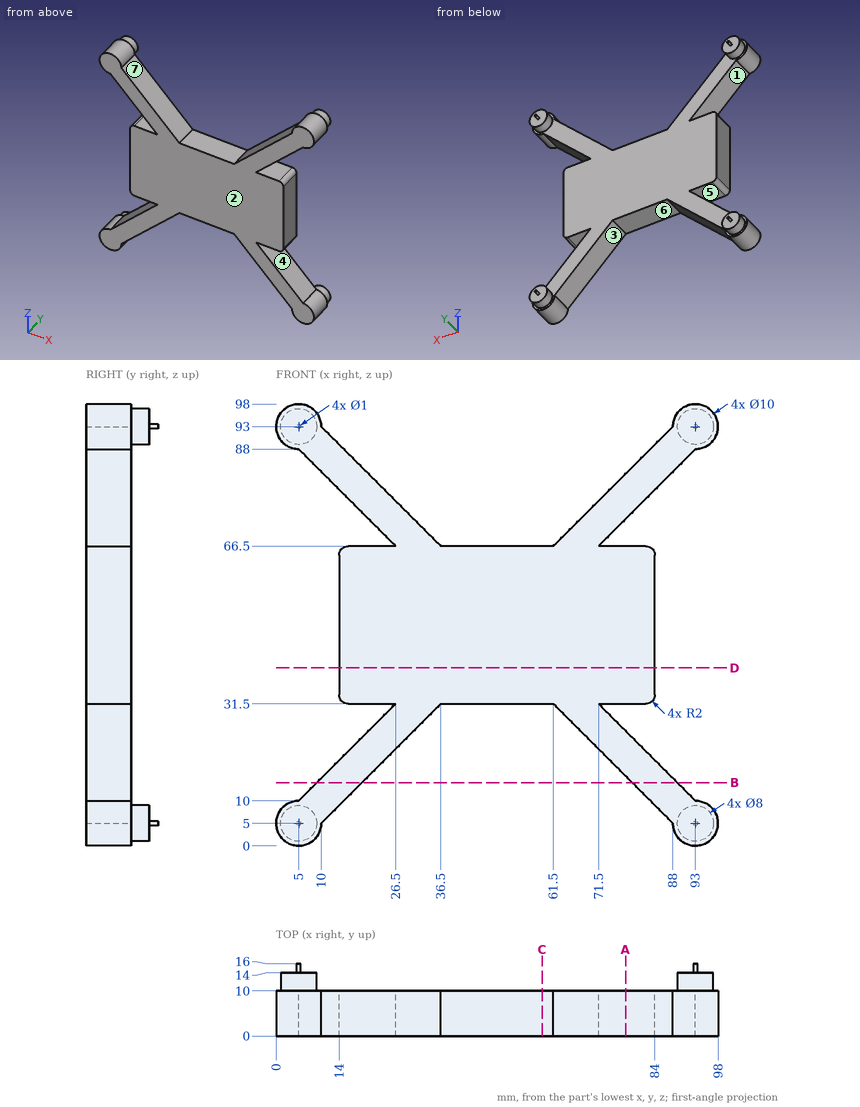
The drawing under review shows one solid part. Ordinate dimensions are in mm from its lowest x, y, z. A direction names the side the tool comes from. Coordinates: 2 decimals unless noted, no trailing zeros. Loops run counter-clockwise (first coordinate to the right, second up) from the corner with the lowest first, then second, coordinate; pieces in that order, holes last. Notation, with made-up numbers: M 89.25,-5.75 L 97.25,-5.75 A14 cw 97.25,17.25 Z; hole C 4,-31 d3. An arc over 180 degrees is marked long. Use one line per item in the form item = value.
(1) Draft analysis for pull direction Z (two halves, no side actions). For the marked faces 1, 2 and 3, state which applies: pulls with the +Z half, pulls with the -Z half, needs draft (parallel to the pull), parting line crosses it, or undercut.
Return value:
face_1 = undercut
face_2 = needs draft
face_3 = pulls with the -Z half
(2) Consider section C-C (x = 59). Write out the cut boundary in (y, z), and give its area (3 significant figures).
Return value:
outline = M 0,31.5 L 10,31.5 L 10,66.5 L 0,66.5 Z
area = 350 mm2
(3) Consider section B-B (z = 14). Write out the cut boundary in (x, y).
Return value:
outline = M 9,0 L 19,0 L 19,10 L 9,10 Z; M 79,0 L 89,0 L 89,10 L 79,10 Z
(4) Consider section A-A (x = 77.5). Write out the cut boundary in (y, z).
Return value:
outline = M 0,15.5 L 10,15.5 L 10,25.5 L 0,25.5 Z; M 0,31.5 L 10,31.5 L 10,66.5 L 0,66.5 Z; M 0,72.5 L 10,72.5 L 10,82.5 L 0,82.5 Z
(5) Consider section D-D (z = 39.5). Write out the cut boundary in (x, y), and give its area (3 significant figures).
Return value:
outline = M 14,0 L 84,0 L 84,10 L 14,10 Z
area = 700 mm2
(6) For the marked faces 4, 5, 6 and 7, list the 3-axis set-ups (+Z, -Z, +X, -X, +Y, -Y) from which the entire face can be reached by the end or side of a thin tool; tool diameter is ignored.
Return value:
face_4 = +X, +Y, -Y
face_5 = -X, +Y, -Y
face_6 = -Z, +Y, -Y
face_7 = +Z, +Y, -Y
(7) Clearance check with flat-ended pins moving along their axes: P1, Ø8, axis at x = 19, z = 86, coming from the +Y side; P2, Ø9, axis at x = 91.5, z = 6, coming from the +Y side; P3, Ø5, axis at x = 51.5, y = 6, coming from the +Z side; P4, Ø1, axis at y = 9.5, z = 64.5, coming from the -X side. State where each tip first meets the part, or that it passes through.
Return value:
P1 = 10
P2 = 16
P3 = 66.5
P4 = 14
(8) For line 1 along Z through (x, y) = (15.5, 7.25); line 2 along X through (y, z) = (3.25, 62); line 3 along X through (y, z) = (5.5, 78.5), list the stretches that pass through material, from the lowest coordinate up. Write a range as from..to.
Return value:
line_1 = 10.5..20.5, 31.56..66.44, 77.5..87.5
line_2 = 14..84
line_3 = 14.5..24.5, 73.5..83.5
